Design review of the part shown in the three views and the two pictorial views. Dimensions are in mm from the part's minimum x, y and z. Round coordinates to 2 decimals unless told otherwise and drop trailing zeros. Order: outer loops, then holes, each group sorted by start corner. A loop starts at its lowest first (then second) coordinate and runs counter-clockwise, first axis right, second up. Notation, with made-up numbers: M -24.75,32 L -17.75,32 A16 cw -17.75,38 Z; hole C -26,-11 d5. An arc over 180 degrees is marked long. Write each question's results on one line, items separated by ' | '. Start each with the question number.
Item 1: Clearance check with flat-ended pins moving along their axes: pin 1 (10 mm diameter, centred on y = 64.5, z = 130.5, fed in from -X); pin 2 (3 mm diameter, centred on x = 84.5, y = 131.5, fed in from -Z). State where each tip first meets the part, or that it passes through.
Item 2: Wall thickness on line 1 (Z direction, x = 30.5, y = 69.5); line 2 (X direction, y = 64.5, z = 130.5): over which ranges is each line inside the solid? List them lowest first. Write a range as [from, to].
Item 3: The part is to be moulded in two halves that separate along X. For the marked faces 1, 2 and 3, say which applies: +X half, -X half, draft (parallel to the pull), parting line (faces both ways), or undercut.
Item 4: Take a section at B-B, the plane z = 81.5. Write out the cut boundary in (x, y), plus the area to 3 significant figures.
Item 5: Take a section at A-A, the plane y = 115. Write out the cut boundary in (x, z).
Item 6: Take a section at C-C, the plane x = 64. Write out the cut boundary in (y, z).
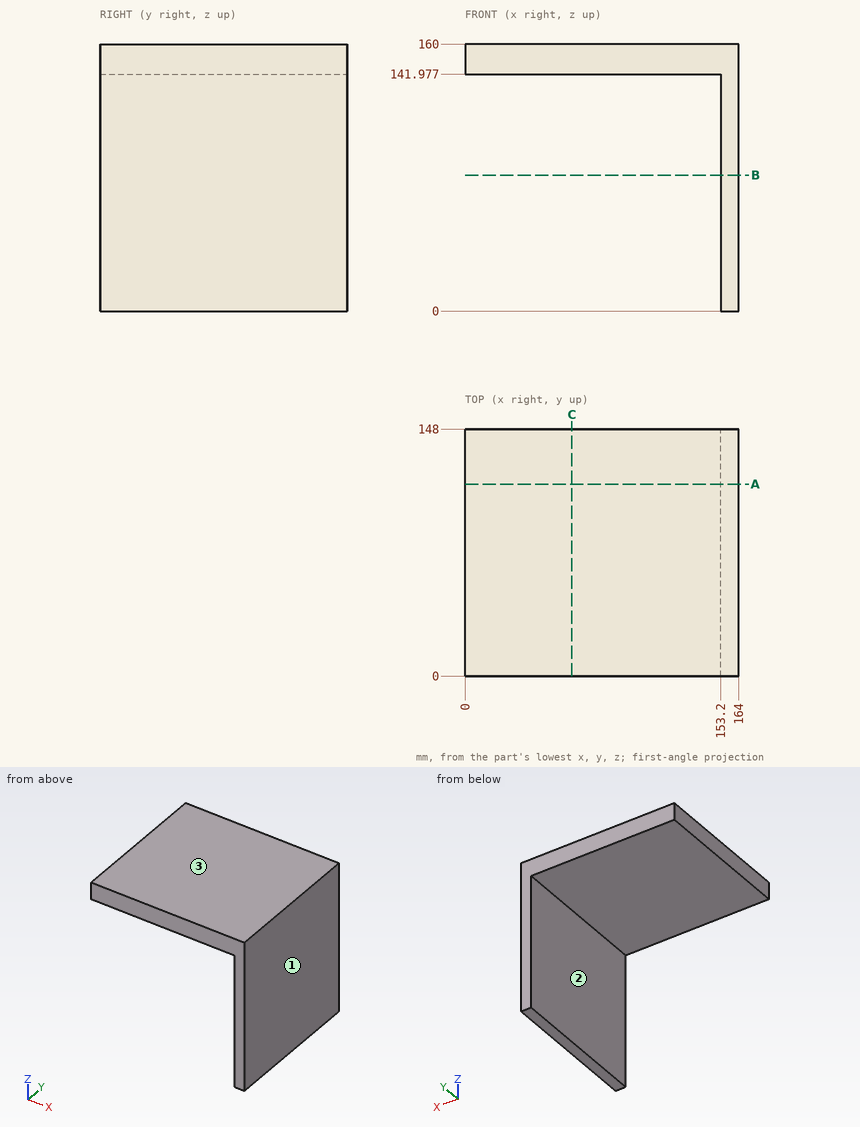
Results list:
1) pin 1: x = 153.2 | pin 2: z = 141.98
2) line 1: [141.98, 160] | line 2: [153.2, 164]
3) face 1: +X half | face 2: -X half | face 3: draft
4) outline: M 153.2,0 L 164,0 L 164,148 L 153.2,148 Z | area: 1,600 mm²
5) outline: M 0,141.98 L 153.2,141.98 L 153.2,0 L 164,0 L 164,160 L 0,160 Z
6) outline: M 0,141.98 L 148,141.98 L 148,160 L 0,160 Z
